Part model, mm, in its own coordinate system. Coordinates: 2 decimals unless noted, no trailing zeros. Write each loop counter-clockwise with the first axis right and the second up, starting at its lowest first coordinate (ties: lowest second). Pieces come first, ordered by that corner, then holes. Notation, with made-up numbers: M 12.5,82 L 25.5,82 A24 ccw 25.5,99 Z; hole C 5.5,-25 d2. An arc over 180 degrees is marked long. Use a Markdown table: item, result. Add a question column.
Q1. Slice it at B-B on x = 4.5. Write the cut outline in (y, z), then the cut area to 3 significant figures.
Q2. Pin check, flat tips, straight feed: pin 1 Ø0.9 at (y, z) = (4, 1.5) entering from -X; pin 2 Ø1 at (x, y) = (0.5, -15) entering from +Z; pin 3 Ø1.6 at (y, z) = (-27.5, 1) entering from +X; pin 4 Ø4.5 at (x, y) = (0, 0) entering from +Z. Stop position of each tip, or through.
Q3. Slice it at A-A on y = -21. Write the cut outline in (x, z).
Q4. Slice it at C-C on x = 11.25. Write the cut outline in (y, z).
Q5. Wall check: L1, parallel to Y at x = 0, z = 0.25; L2, parallel to Y at x = 0.25, z = 2; L3, parallel to Z at x = 17.5, y = 1.5. Give the ranges that are in metal, low to high. Write a range as from..to.
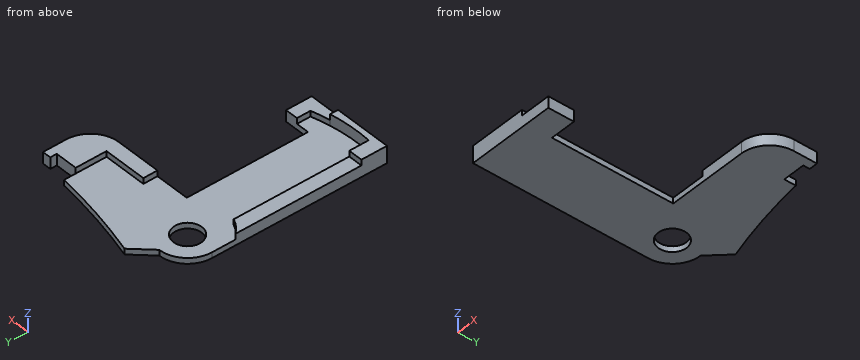
from build123d import *

# Parameters (mm, degrees)
EXTRUDE_3_DEPTH = 3
EXTRUDE_4_DEPTH = 2
SKETCH_1_8_R    = 2.5
EXTRUDE_5_DEPTH = 1


with BuildPart() as part:
    # Sketch 1 → Extrude 3 (new body)
    with BuildSketch(Plane.XY):
        with BuildLine():
            Line((-2.5, -26.437677825), (-5, -26.437677825))
            Line((-5, -26.437677825), (-5, -30.96175738))
            Line((-5, -30.96175738), (5.076141326, -30.96175738))
            Line((5.076141326, -30.96175738), (5.076141326, -29.54601506))
            ThreePointArc((5.076141326, -29.54601506), (1.298498135, -29.950761581), (-2.5, -29.874474333))
            Line((-2.5, -29.874474333), (-2.5, -26.437677825))
        make_face()
    extrude(amount=EXTRUDE_3_DEPTH)

    # Sketch 1_7 → Extrude 4 (add)
    with BuildSketch(Plane.XY):
        with BuildLine():
            Line((23.502499093, 2.950728465), (19.6, 2.950728465))
            Line((19.6, 2.950728465), (19.6, -2.5))
            Line((19.6, -2.5), (12.023157318, -2.5))
            Line((12.023157318, -2.5), (12.023157318, -5))
            Line((12.023157318, -5), (20, -5))
            ThreePointArc((20, -5), (23.535533906, -3.535533906), (25, 0))
            Line((25, 0), (25, 4.09591659))
            Line((25, 4.09591659), (23.502499093, 4.09591659))
            Line((23.502499093, 4.09591659), (23.502499093, 2.950728465))
        make_face()
        with BuildLine():
            ThreePointArc((-2.5, -6), (-3.862002616, -5.228282299), (-5, -4.153311931))
            Line((-5, -4.153311931), (-5, -26.437677825))
            Line((-5, -26.437677825), (-2.5, -26.437677825))
            Line((-2.5, -26.437677825), (-2.5, -6))
        make_face()
        with BuildLine():
            Line((5.076141326, -29.54601506), (5.076141326, -30.96175738))
            Line((5.076141326, -30.96175738), (10.508252403, -30.96175738))
            Line((10.508252403, -30.96175738), (10.508252403, -26.437677825))
            Line((10.508252403, -26.437677825), (8.264928228, -26.437677825))
            Line((8.264928228, -26.437677825), (8.264928228, -28.81709871))
            ThreePointArc((8.264928228, -28.81709871), (6.680483813, -29.225080884), (5.076141326, -29.54601506))
        make_face()
    extrude(amount=EXTRUDE_4_DEPTH)


with BuildPart() as extrude_4_piece_1:
    # of the separate pieces the step leaves, piece 1, a body of its own (extrude_4_pieces)
    add(part.part.solids().sort_by_distance((-2.5, -29.874474333, 0))[0])



with BuildPart() as extrude_4_piece_2:
    # of the separate pieces the step leaves, piece 2, a body of its own (extrude_4_pieces)
    add(part.part.solids().sort_by_distance((23.502499093, 2.950728465, 0))[0])


with BuildPart() as extrude_4_piece_1_1:
    add(extrude_4_piece_1.part)

    add(extrude_4_piece_2.part)  # Extrude 5 merges Extrude 4 piece 2
    # Sketch 1_8 → Extrude 5 (add)
    with BuildSketch(Plane.XY):
        with BuildLine():
            Line((3.231912185, 8.38327913), (0, 5))
            ThreePointArc((0, 5), (-3.535533906, 3.535533906), (-5, 0))
            Line((-5, 0), (-5, -4.153311931))
            ThreePointArc((-5, -4.153311931), (-3.862002616, -5.228282299), (-2.5, -6))
            Line((-2.5, -6), (-2.5, -29.874474333))
            ThreePointArc((-2.5, -29.874474333), (2.93054776, -29.83531643), (8.264928228, -28.81709871))
            Line((8.264928228, -28.81709871), (8.264928228, -26.437677825))
            Line((8.264928228, -26.437677825), (5.994868924, -26.437677825))
            Line((5.994868924, -26.437677825), (5.994868924, -5))
            Line((5.994868924, -5), (12.023157318, -5))
            Line((12.023157318, -5), (12.023157318, -2.5))
            Line((12.023157318, -2.5), (19.6, -2.5))
            Line((19.6, -2.5), (19.6, 5))
            ThreePointArc((19.6, 5), (11.347380216, 6.359873864), (3.231912185, 8.38327913))
        make_face()
        Circle(SKETCH_1_8_R, mode=Mode.SUBTRACT)
    extrude(amount=EXTRUDE_5_DEPTH)


solid = extrude_4_piece_1_1.part
Recorded:
| question | item | result |
|---|---|---|
| 1 | outline | M -30.96,0 L 8.02,0 L 8.02,1 L -29.64,1 L -29.64,3 L -30.96,3 Z |
| 1 | area | 41.6 mm² |
| 2 | pin 1 | x = 23.5 |
| 2 | pin 2 | z = 1 |
| 2 | pin 3 | x = 10.51 |
| 2 | pin 4 | through |
| 3 | outline | M -5,0 L 5.99,0 L 5.99,1 L -2.5,1 L -2.5,2 L -5,2 Z |
| 4 | outline | M -5,0 L 6.38,0 L 6.38,1 L -5,1 Z |
| 5 | L1 | -30.96..-2.5, 2.5..5 |
| 5 | L2 | -30.96..-29.98 |
| 5 | L3 | 0..1 |
